Source: CAD feature listing. Evaluate the final solid. Frame: model axes, mm. Coordinates: 2 decimals unless noted, no trailing zeros. Write each loop counter-clockwise with the first axis right and the second up, starting at its lowest first coordinate (ties: lowest second). Pieces come first, ordered by that corner, then holes. Notation, with made-up numbers: (62.25, -23) - (87.25, -23) arc R13 ccw to (87.25, -14) - close; hole circle Ø3 at (-26, 9). An arc over 180 degrees is marked (long way). One line per question, with ' | ' between items. Start each with the question number.
Q1. Cut plane D-D, the plane x = 114.5. Return loops of the section in (y, z), plus the area to 3 significant figures.
Q2. Contact query for flat-ended pins moving along their axis: P1, Ø3, axis at x = 123, z = 2.5, coming from the +Y side; P2, Ø1, axis at y = 25.5, z = 2, coming from the +X side (3 decimals); P3, Ø1.5, axis at x = 9.5, z = 2, coming from the -Y side. Output: stop coordinate, or through.
Q3. Line query: line 1 (X direction, y = 29.5, z = 6.25) (3 decimals); line 2 (X direction, y = 25.5, z = 3.25) (3 decimals); line 3 (X direction, y = 12, z = 3.5) (3 decimals). Output: solid intervals per line, ascending.
Q4. Cut plane A-A, the plane y = 3. Return loops of the section in (x, z) (3 decimals), plus the area to 3 significant figures.
Q5. Cut plane C-C, the plane y = 14. Return loops of the section in (x, z) (3 decimals), plus the area to 3 significant figures.
Q6. Cut plane B-B, the plane y = 29. Return loops of the section in (x, z) (3 decimals), plus the area to 3 significant figures.
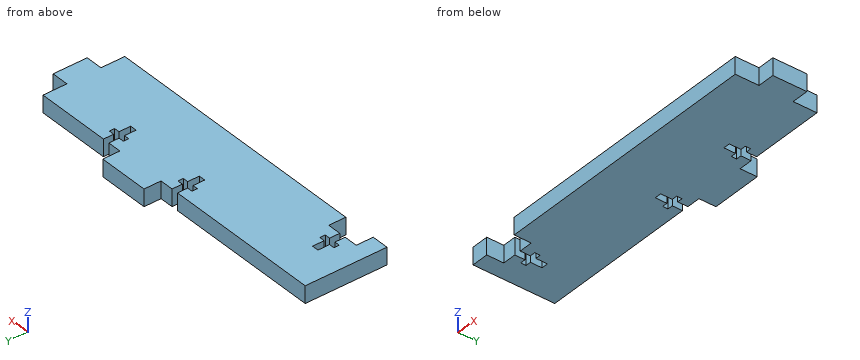
```python
from build123d import *

# Parameters (mm, degrees)
BOSS_EXTRUDE1_DEPTH = 6.35
SKETCH2_W           = 12.7
SKETCH2_H           = 6.35
CUT_EXTRUDE1_DEPTH  = 7.35
CUT_EXTRUDE5_DEPTH  = 7.35


with BuildPart() as part:
    # Sketch1 → Boss-Extrude1 (new body)
    with BuildSketch(Plane.XY):
        Polygon((66.675, 30.48), (0, 30.48), (0, 0), (121.285, 0), (121.285, 8.89), (127.635, 8.89), (127.635, 21.59), (121.285, 21.59), (121.285, 30.48), (85.725, 30.48), (85.725, 36.83), (66.675, 36.83), align=None)
    extrude(amount=BOSS_EXTRUDE1_DEPTH)

    # Sketch2 → Cut-Extrude1 (cut, through all)
    with BuildSketch(Plane.XY.offset(6.35)):
        with Locations((12.7, 3.175)):
            Rectangle(SKETCH2_W, SKETCH2_H)
    extrude(amount=-CUT_EXTRUDE1_DEPTH, mode=Mode.SUBTRACT)

    # Sketch5 → Cut-Extrude5 (cut, through all)
    with BuildSketch(Plane.XY.offset(6.35)):
        Polygon((61.575, 30.48), (59.075, 30.48), (59.075, 26.67), (57.075, 26.67), (57.075, 24.67), (59.075, 24.67), (59.075, 20.32), (61.575, 20.32), (61.575, 24.67), (63.575, 24.67), (63.575, 26.67), (61.575, 26.67), align=None)
        Polygon((90.825, 26.67), (88.825, 26.67), (88.825, 24.67), (90.825, 24.67), (90.825, 20.32), (93.325, 20.32), (93.325, 24.67), (95.325, 24.67), (95.325, 26.67), (93.325, 26.67), (93.325, 30.48), (90.825, 30.48), align=None)
        Polygon((11.45, 10.16), (11.45, 6.35), (13.95, 6.35), (13.95, 10.16), (15.95, 10.16), (15.95, 12.16), (13.95, 12.16), (13.95, 16.51), (11.45, 16.51), (11.45, 12.16), (9.45, 12.16), (9.45, 10.16), align=None)
    extrude(amount=-CUT_EXTRUDE5_DEPTH, mode=Mode.SUBTRACT)


solid = part.part
```
Reply:
1) outline: (0, 0) - (30.48, 0) - (30.48, 6.35) - (0, 6.35) - close | area: 194 mm^2
2) P1: stops at y = 21.59 | P2: stops at x = 121.285 | P3: stops at y = 6.35
3) line 1: x = 0 to 59.075, 61.575 to 90.825, 93.325 to 121.285 | line 2: x = 0 to 57.075, 63.575 to 88.825, 95.325 to 121.285 | line 3: x = 0 to 9.45, 15.95 to 127.635
4) outline: (0, 0) - (6.35, 0) - (6.35, 6.35) - (0, 6.35) - close; (19.05, 0) - (121.285, 0) - (121.285, 6.35) - (19.05, 6.35) - close | area: 690 mm^2
5) outline: (0, 0) - (11.45, 0) - (11.45, 6.35) - (0, 6.35) - close; (13.95, 0) - (127.635, 0) - (127.635, 6.35) - (13.95, 6.35) - close | area: 795 mm^2
6) outline: (0, 0) - (59.075, 0) - (59.075, 6.35) - (0, 6.35) - close; (61.575, 0) - (90.825, 0) - (90.825, 6.35) - (61.575, 6.35) - close; (93.325, 0) - (121.285, 0) - (121.285, 6.35) - (93.325, 6.35) - close | area: 738 mm^2
